The model under review builds one solid part; all positions refer to its coordinate system, in mm. A direction names the side the tool comes from. Round coordinates to 2 decimals unless told otherwise and drop trailing zeros.
Item 1: Machinability: for faces 1 (the face through (127, 3, -13)), 2 (the face through (2.897, 3.219, -259.284)), which of the approach directions +Z, -Z, +X, -X, +Y, -Y give a long, thin tool a straight path to every point of the face, cutting with its end or side? Answer none if there is none.
Item 2: To check wall thickness, follow L1, parallel to X at y = 5, z = -114.3; L2, parallel to X at y = 3, z = -250.5; L3, parallel to Z at x = 128, y = 4.5. State the ranges of each line that lie inside material, in increasing order.
Item 3: Draft analysis for pull direction X (two halves, no side actions). For faces 3 (the face through (0, 3, -129)), 4 (the face through (130, 3, -16.388)), 5 (the face through (149.345, 3.219, -2.897)), state which applies: +X half, -X half, draft (parallel to the pull), parting line (faces both ways), or undercut.
Item 4: Clearance check with flat-ended pins moving along their axes: pin 1 Ø3.5 at (x, z) = (41.91, -38.1) entering from -Y; pin 2 Ø2.5 at (x, z) = (110.49, -224.24) entering from -Y. State where each tip first meets the part, or that it passes through.
```python
from build123d import *

# Parameters (mm, degrees)
SKETCH3_W           = 152.4
SKETCH3_H           = 262.339276313
SKETCH3_R           = 1.4224
SKETCH3_W_2         = 6.35
SKETCH3_H_2         = 6.35
BOSS_EXTRUDE1_DEPTH = 6.35
FILLET1_R           = 10.16


with BuildPart() as part:
    # Sketch3 → Boss-Extrude1 (new body)
    with BuildSketch(Plane(origin=(0, 0, 0), x_dir=(1, 0, 0), z_dir=(0, 1, 0))):
        with Locations((76.2, 131.169638157)):
            Rectangle(SKETCH3_W, SKETCH3_H)
        with Locations(Location((41.91, 38.1, 0), (0, 0, 270))):
            Circle(SKETCH3_R, mode=Mode.SUBTRACT)
        with Locations(Location((41.91, 114.3, 0), (0, 0, 270))):
            Circle(SKETCH3_R, mode=Mode.SUBTRACT)
        with Locations(Location((110.49, 114.3, 0), (0, 0, 90))):
            Circle(SKETCH3_R, mode=Mode.SUBTRACT)
        with Locations(Location((110.49, 38.1, 0), (0, 0, 90))):
            Circle(SKETCH3_R, mode=Mode.SUBTRACT)
        with Locations(Location((54.61, 151.157668748, 0), (0, 0, 270))):
            Circle(SKETCH3_R, mode=Mode.SUBTRACT)
        with Locations(Location((54.61, 219.737668748, 0), (0, 0, 270))):
            Circle(SKETCH3_R, mode=Mode.SUBTRACT)
        with Locations(Location((97.79, 151.157668748, 0), (0, 0, 90))):
            Circle(SKETCH3_R, mode=Mode.SUBTRACT)
        with Locations(Location((97.79, 219.737668748, 0), (0, 0, 90))):
            Circle(SKETCH3_R, mode=Mode.SUBTRACT)
        with Locations(Location((97.79, 42.601607565, 0), (0, 0, 270))):
            Circle(SKETCH3_R, mode=Mode.SUBTRACT)
        with Locations(Location((97.79, 111.181607565, 0), (0, 0, 270))):
            Circle(SKETCH3_R, mode=Mode.SUBTRACT)
        with Locations(Location((54.61, 111.181607565, 0), (0, 0, 90))):
            Circle(SKETCH3_R, mode=Mode.SUBTRACT)
        with Locations(Location((54.61, 42.601607565, 0), (0, 0, 90))):
            Circle(SKETCH3_R, mode=Mode.SUBTRACT)
        with Locations(Location((110.49, 148.039276313, 0), (0, 0, 270))):
            Circle(SKETCH3_R, mode=Mode.SUBTRACT)
        with Locations(Location((110.49, 224.239276313, 0), (0, 0, 270))):
            Circle(SKETCH3_R, mode=Mode.SUBTRACT)
        with Locations(Location((41.91, 224.239276313, 0), (0, 0, 90))):
            Circle(SKETCH3_R, mode=Mode.SUBTRACT)
        with Locations(Location((41.91, 148.039276313, 0), (0, 0, 90))):
            Circle(SKETCH3_R, mode=Mode.SUBTRACT)
        with Locations((22.225, 13.212735966)):
            Rectangle(SKETCH3_W_2, SKETCH3_H_2, mode=Mode.SUBTRACT)
        with Locations((130.175, 13.212735966)):
            Rectangle(SKETCH3_W_2, SKETCH3_H_2, mode=Mode.SUBTRACT)
        with Locations((130.175, 249.126540348)):
            Rectangle(SKETCH3_W_2, SKETCH3_H_2, mode=Mode.SUBTRACT)
        with Locations((22.225, 249.126540348)):
            Rectangle(SKETCH3_W_2, SKETCH3_H_2, mode=Mode.SUBTRACT)
    extrude(amount=BOSS_EXTRUDE1_DEPTH)

    # Fillet1
    fillet1_edges = [part.edges().sort_by_distance(p)[0] for p in [
        (0, 3.175, -262.339276313),
        (152.4, 3.175, -262.339276313),
        (152.4, 3.175, 0),
        (0, 3.175, 0),
    ]]
    fillet(fillet1_edges, radius=FILLET1_R)


solid = part.part
```
Numbers:
1. face 1: +Y, -Y
1. face 2: -Z, -X, +Y, -Y
2. L1: x = 0 to 40.49, 43.33 to 109.07, 111.91 to 152.4
2. L2: x = 0 to 19.05, 25.4 to 127, 133.35 to 152.4
2. L3: z = -262.34 to -252.3, -245.95 to -16.39, -10.04 to 0
3. face 3: -X half
3. face 4: undercut
3. face 5: +X half
4. pin 1: stops at y = 0
4. pin 2: passes through
